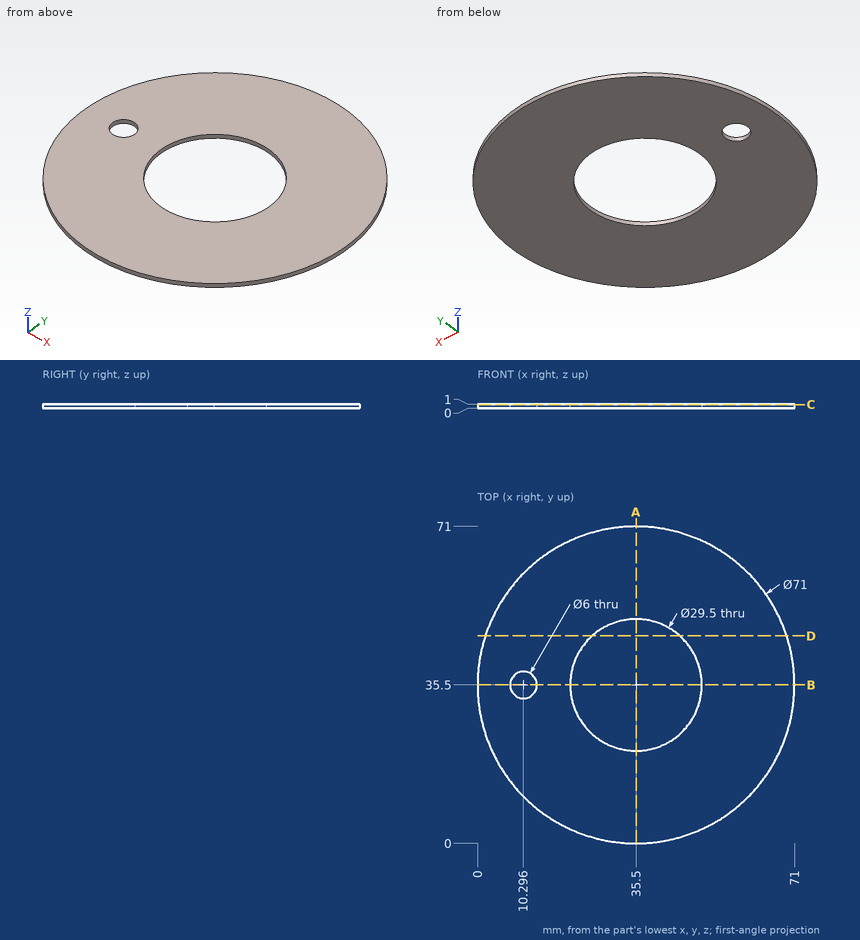
For this review, use the dimensioned drawing (mm, ordinates from the lowest corner) and the shaded views. Give positions to 0.01 mm unless a question says otherwise; leave off trailing zeros. Order: outer loops, then holes, each group sorted by start corner. A loop starts at its lowest first (then second) coordinate and runs counter-clockwise, first axis right, second up. Notation, with made-up numbers: (6, 8.25) - (38, 8.25) arc R16 ccw to (38, 35.25) - close; hole circle Ø7 at (-4.5, 40). An arc over 180 degrees is marked (long way). Use a Markdown table: item, result. Add a question column.
(1) Add section C-C on z = 0.85. Give the boundary of the cut face in (x, y).
(2) Add section A-A on x = 35.5. Give the boundary of the cut face in (y, z).
(3) Add section B-B on y = 35.5. Give the boundary of the cut face in (x, z).
(4) Wall thickness on probe 1 along Y at (x, z) = (35.5, 0.45); probe 2 along X at (y, z) = (25.5, 0.9) (1 decimal); probe 3 along Y at (x, z) = (22, 0.6) (1 decimal): over which ranges is each line inside the solid? List them lowest first. Write a range as [from, to].
(5) Add section D-D on y = 46.5. Give the boundary of the cut face in (x, z).
Report:
| question | item | result |
|---|---|---|
| 1 | outline | circle Ø71 at (35.5, 35.5); hole circle Ø6 at (10.3, 35.5); hole circle Ø29.5 at (35.5, 35.5) |
| 2 | outline | (0, 0) - (20.75, 0) - (20.75, 1) - (0, 1) - close; (50.25, 0) - (71, 0) - (71, 1) - (50.25, 1) - close |
| 3 | outline | (0, 0) - (7.3, 0) - (7.3, 1) - (0, 1) - close; (13.3, 0) - (20.75, 0) - (20.75, 1) - (13.3, 1) - close; (50.25, 0) - (71, 0) - (71, 1) - (50.25, 1) - close |
| 4 | probe 1 | y = [0, 20.75], [50.25, 71] |
| 4 | probe 2 | x = [1.4, 24.7], [46.3, 69.6] |
| 4 | probe 3 | y = [2.7, 29.6], [41.4, 68.3] |
| 5 | outline | (1.75, 0) - (25.67, 0) - (25.67, 1) - (1.75, 1) - close; (45.33, 0) - (69.25, 0) - (69.25, 1) - (45.33, 1) - close |
